Autodesk Inventor part; units mm, degrees
ref_plane "YZ Plane" through (0, 0, 0) normal (1, 0, 0) x (0, 1, 0)
ref_plane "XZ Plane" through (0, 0, 0) normal (0, 1, 0) x (-1, 0, 0)
ref_plane "XY Plane" through (0, 0, 0) normal (0, 0, 1) x (1, 0, 0)
sketch "Sketch1" plane through (0, 0, 0) normal (1, 0, 0) x (0, 1, 0)
  circle A0 centre (0, 0) radius 3
  dimension "d0" = 6
extrude "Extrusion1" add sketch "Sketch1" along normal blind 3
chamfer "Chamfer1" distance 0.5 angle 45 1 edges at (0, -3, 0)
sketch "Sketch2" plane through (3, 0, 0) normal (1, 0, 0) x (0, 0, -1)
  circle A0 centre (0, 0) radius 1.5
  dimension "d6" = 3
extrude "Extrusion2" add sketch "Sketch2" along normal blind 17
chamfer "Chamfer2" distance 0.5 angle 45 1 edges at (20, 0, 1.5)
thread "Thread1"
properties part number "Reverse Gear LInk Stud" material "Steel"
Input: part model. Units: mm. Frame: model coordinates. A direction names the side the tool comes from. Coordinates: 2 decimals unless noted, no trailing zeros. Write each loop counter-clockwise with the first axis right and the second up, starting at its lowest first coordinate (ties: lowest second). Pieces come first, ordered by that corner, then holes.
1) Set-up query: faces 1 (the cylindrical face through (11.13, -0.07, 1.5)), 2 (the cylindrical face through (2, -3, 0)). Return all of +Z, -Z, +X, -X, +Y, -Y with unobstructed straight access to the full face (end or side cutting, diameter ignored); none if empty.
2) Material intervals for line 1 along X through (y, z) = (2, -1.2); line 2 along Y through (x, z) = (2.25, 0.15); line 3 along Y through (x, z) = (5.75, 0.7), sorted ascending.
3) Section A-A on y = 0. Output: boundary loops of the cut face in (x, z).
4) Section C-C on x = 8.25. Output: boundary loops of the cut face in (y, z).
5) Pin query (flat end, axial travel): pin 1 Ø2 at (x, y) = (3.5, -1.5) entering from -Z. Return the tip coordinate at first contact, or that it passes through.
Check result:
1. face 1: +X
1. face 2: +X, -X
2. line 1: x = 0 to 3
2. line 2: y = -3 to 3
2. line 3: y = -1.33 to 1.33
3. outline: (0, -2.5) - (0.5, -3) - (3, -3) - (3, -1.5) - (19.5, -1.5) - (20, -1) - (20, 1) - (19.5, 1.5) - (3, 1.5) - (3, 3) - (0.5, 3) - (0, 2.5) - close
4. outline: circle Ø3 at (0, 0)
5. pin 1: stops at z = -2.93
